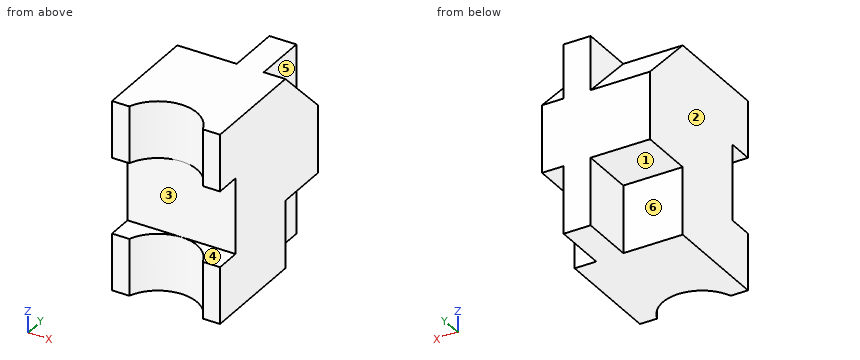
from build123d import *

# Parameters (mm, degrees)
EXTRUDE_1_DEPTH     = 70
SKETCH_2_W          = 28
SKETCH_2_H          = 9.5
CUT_EXTRUDE_1_DEPTH = 87.02325267
SKETCH_3_W          = 25
SKETCH_3_H          = 20
CUT_EXTRUDE_2_DEPTH = 8
CUT_EXTRUDE_START   = -18
SKETCH_3_2_W        = 25
SKETCH_3_2_H        = 20
CUT_EXTRUDE_3_DEPTH = 69.02325267


with BuildPart() as part:
    # Sketch 1 → Extrude 1 (new body)
    with BuildSketch(Plane.XY):
        with BuildLine():
            Line((-7, 30), (-20, -10))
            Line((-20, -10), (-20, -30))
            Line((-20, -30), (-13.610657589, -30))
            ThreePointArc((-13.610657589, -30), (0, -20.5), (13.610657589, -30))
            Line((13.610657589, -30), (20, -30))
            Line((20, -30), (20, 30))
            Line((20, 30), (-7, 30))
        make_face()
        Polygon((-20, 30), (-20, -10), (-7, 30), align=None)
    extrude(amount=EXTRUDE_1_DEPTH)

    # Sketch 2 → Cut-Extrude 1 (cut, through all)
    with BuildSketch(Plane.ZY.offset(20)):
        with Locations((35, -25.25)):
            Rectangle(SKETCH_2_W, SKETCH_2_H)
    extrude(amount=-CUT_EXTRUDE_1_DEPTH, mode=Mode.SUBTRACT)

    # Sketch 3 → Cut-Extrude 2 (cut)
    with BuildSketch(Plane(origin=(20, 0, 0), x_dir=(0, 0, -1), z_dir=(1, 0, 0))):
        Polygon((-70, 30), (-70, 10), (-50, 30), align=None)
        with Locations((-12.5, 20)):
            Rectangle(SKETCH_3_W, SKETCH_3_H)
    extrude(amount=-CUT_EXTRUDE_2_DEPTH, mode=Mode.SUBTRACT)

    # Sketch 3_2 → Cut-Extrude 3 (cut, through all)
    with BuildSketch(Plane(origin=(20, 0, 0), x_dir=(0, 0, -1), z_dir=(1, 0, 0)).offset(CUT_EXTRUDE_START)):
        Polygon((-70, 30), (-70, 10), (-50, 30), align=None)
        with Locations((-12.5, 20)):
            Rectangle(SKETCH_3_2_W, SKETCH_3_2_H)
    extrude(amount=-CUT_EXTRUDE_3_DEPTH, mode=Mode.SUBTRACT)


solid = part.part
Build history of the part. All positions in model axes, mm. Face numbers are marked on the shaded views. A direction names the side the tool comes from. Round coordinates to 2 decimals unless told otherwise and drop trailing zeros. Loops run counter-clockwise (first coordinate to the right, second up) from the corner with the lowest first, then second, coordinate; pieces in that order, holes last. Notation, with made-up numbers: (53, 4.5) -> (91, 4.5) arc R15 cw to (91, 17.5) -> close; hole circle Ø3 at (-12, 59). An arc over 180 degrees is marked (long way). One line per item, written item: value. Start each with the question number.
Q1. Cut at C-C on y = -24. List the corners of the cut face in (x, z), plus the area to 3 significant figures.
Q2. Cut at B-B on z = 56. List the corners of the cut face in (x, y).
Q3. Probe line 1 along Z through (x, y) = (16, -24); line 2 along Y through (x, z) = (5, 33.5); line 3 along Y through (x, z) = (-3, 22.5). List the from-to ranges inside material, lowest first.
Q4. Cut at D-D on x = -10.5. List the corners of the cut face in (y, z).
Q5. 3-axis set-ups, long thin cutter, end or side, ignore diameter. For the marked faces 4, 5 and 6: which of +Z, -Z, +X, -X, +Y, -Y reach the whole face in a straight line?
Q6. Two-plate mould, pull along Z, no slides. Class the marked faces 1, 2 and 3: released by +Z, released by -Z, zero draft, split by the parting line, or undercut.
Q7. Cut at A-A on y = 18.5. List the corners of the cut face in (x, z), plus the area to 4 significant figures.
Q8. Drop flat-ended pins along their axis: pin 1 Ø11 at (x, z) = (-7, 14.5) entering from +Y; pin 2 Ø12 at (x, z) = (-16, 38) entering from -Y; pin 3 Ø16 at (y, z) = (25, 10) entering from +X. Give the stop position or say it passes through.
Computed:
1. outline: (-20, 0) -> (-9.45, 0) -> (-9.45, 21) -> (-20, 21) -> close; (-20, 49) -> (-9.45, 49) -> (-9.45, 70) -> (-20, 70) -> close; (9.45, 0) -> (20, 0) -> (20, 21) -> (9.45, 21) -> close; (9.45, 49) -> (20, 49) -> (20, 70) -> (9.45, 70) -> close
1. area: 886 mm²
2. outline: (-20, -30) -> (-13.61, -30) arc R14.5 cw to (13.61, -30) -> (20, -30) -> (20, 24) -> (12, 24) -> (12, 30) -> (2, 30) -> (2, 24) -> (-20, 24) -> close
3. line 1: 0 to 21, 49 to 70
3. line 2: -20.5 to 30
3. line 3: -20.5 to 10
4. outline: (-25, 0) -> (10, 0) -> (10, 25) -> (30, 25) -> (30, 50) -> (10, 70) -> (-25, 70) -> (-25, 49) -> (-20.5, 49) -> (-20.5, 21) -> (-25, 21) -> close
5. face 4: +X, -X, -Y
5. face 5: +Z, +X, +Y
5. face 6: -Z, -X, +Y
6. face 1: released by -Z
6. face 2: zero draft
6. face 3: undercut
7. outline: (-20, 25) -> (2, 25) -> (2, 0) -> (12, 0) -> (12, 25) -> (20, 25) -> (20, 61.5) -> (12, 61.5) -> (12, 70) -> (2, 70) -> (2, 61.5) -> (-20, 61.5) -> close
7. area: 1,795 mm²
8. pin 1: y = 10
8. pin 2: y = -20.5
8. pin 3: x = 12
